Geometry: final body of the model. Coordinates: model frame, mm. A direction names the side the tool comes from. Give positions to 0.01 mm unless a question says otherwise; leave off trailing zeros. Loops run counter-clockwise (first coordinate to the right, second up) from the corner with the lowest first, then second, coordinate; pieces in that order, holes last. Notation, with made-up numbers: M 18,39 L 26,39 A23 ccw 26,69 Z; hole C -32,-28.75 d1. An arc over 180 degrees is marked long. Put each result on its own line as item: value.
```python
from build123d import *

# Parameters (mm, degrees)
ESQUISSE1_R                  = 0.85
BOSS_EXTRU_1_DEPTH           = 4
ESQUISSE2_W                  = 5
ESQUISSE2_H                  = 11.5
BOSS_EXTRU_2_DEPTH           = 21
ESQUISSE3_R                  = 1.4
ENL_V_MAT_EXTRU_1_DEPTH      = 93.33964479
CONG_1_R                     = 5
BOSS_EXTRU_3_DEPTH           = 3
BOSS_EXTRU_4_DEPTH           = 25
ESQUISSE6_R                  = 1.2
ENL_V_MAT_EXTRU_2_DEPTH      = 84.712364678
BOSS_EXTRU_6_DEPTH           = 4.5
BOSS_EXTRU_6_DEPTH_BACK      = 4
ESQUISSE9_R                  = 24
ESQUISSE9_R_2                = 21
BOSS_EXTRU_7_DEPTH           = 7
ENL_V_MAT_EXTRU_3_DEPTH      = 87.997255704
ENL_V_MAT_EXTRU_3_DEPTH_BACK = 87.997255704
ESQUISSE11_R                 = 0.9
ENL_V_MAT_EXTRU_4_DEPTH      = 87.997255704
ENL_V_MAT_EXTRU_4_DEPTH_BACK = 87.997255704
ESQUISSE12_R                 = 0.9


with BuildPart() as part:
    # Esquisse1 → Boss.-Extru.1 (new body)
    with BuildSketch(Plane.XY):
        Polygon((15.5, 18), (-15.5, 18), (-72.6, 3.278696541), (-72.6, -18), (-67.6, -18), (-67.6, -6), (-45, -6), (-45, -18), (45, -18), (45, -6), (67.6, -6), (67.6, -18), (72.6, -18), (72.6, 3.278696541), align=None)
        with Locations((-42.5, -12)):
            Circle(ESQUISSE1_R, mode=Mode.SUBTRACT)
        with Locations((-70.1, -12)):
            Circle(ESQUISSE1_R, mode=Mode.SUBTRACT)
        with Locations(Location((42.5, -12, 0), (0, 0, 180))):
            Circle(ESQUISSE1_R, mode=Mode.SUBTRACT)
        with Locations(Location((70.1, -12, 0), (0, 0, 180))):
            Circle(ESQUISSE1_R, mode=Mode.SUBTRACT)
    extrude(amount=BOSS_EXTRU_1_DEPTH)

    # Esquisse2 → Boss.-Extru.2 (add)
    with BuildSketch(Plane(origin=(0, 0, 0), x_dir=(-1, 0, 0), z_dir=(0, 0, -1))):
        with Locations((-13, 12.25)):
            Rectangle(ESQUISSE2_W, ESQUISSE2_H)
        with Locations((13, 12.25)):
            Rectangle(ESQUISSE2_W, ESQUISSE2_H)
    extrude(amount=BOSS_EXTRU_2_DEPTH)

    # Esquisse3 → Enlèv. mat.-Extru.1 (cut, through all)
    with BuildSketch(Plane.ZY.offset(15.5)):
        with Locations((-6.49, 12.25)):
            Circle(ESQUISSE3_R)
        with Locations((-14.49, 12.25)):
            Circle(ESQUISSE3_R)
    extrude(amount=-ENL_V_MAT_EXTRU_1_DEPTH, mode=Mode.SUBTRACT)

    # Congé1
    cong_1_edges = [part.edges().sort_by_distance(p)[0] for p in [
        (-15.5, 12.25, 0),
        (15.5, 12.25, 0),
    ]]
    fillet(cong_1_edges, radius=CONG_1_R)

    # Esquisse4 → Boss.-Extru.3 (add)
    with BuildSketch(Plane.XZ.offset(-6.5)):
        Polygon((-15.5, -10.5), (-39.70316927, -7.340935878), (-46.787327396, 0), (-10.5, 0), (-10.5, -10.5), align=None)
        Polygon((15.5, -10.5), (10.5, -10.5), (10.5, 0), (46.787327396, 0), (39.70316927, -7.340935878), align=None)
    extrude(amount=-BOSS_EXTRU_3_DEPTH)

    # Esquisse5 → Boss.-Extru.4 (add, through all)
    with BuildSketch(Plane.XY.offset(4)):
        Polygon((-15.466226842, 23), (-15.466226842, 18), (15.466226842, 18), (15.466226842, 23), (7.816226842, 23), (7.816226842, 28), (10.316226842, 28), (10.316226842, 30.5), (4.816226842, 30.5), (4.816226842, 26), (-4.816226842, 26), (-4.816226842, 30.5), (-10.316226842, 30.5), (-10.316226842, 28), (-7.816226842, 28), (-7.816226842, 23), align=None)
    extrude(amount=-BOSS_EXTRU_4_DEPTH)

    # Esquisse6 → Enlèv. mat.-Extru.2 (cut, through all)
    with BuildSketch(Plane.XZ.offset(-18)):
        with Locations(Location((0, -5.25, 0), (0, 0, 270))):
            Circle(ESQUISSE6_R)
        with Locations(Location((0, -15.7500125, 0), (0, 0, 270))):
            Circle(ESQUISSE6_R)
    extrude(amount=-ENL_V_MAT_EXTRU_2_DEPTH, mode=Mode.SUBTRACT)

    # Esquisse9 → Boss.-Extru.6 (add, two sides: drawn at the far end of the back side and taken through both)
    with BuildSketch(Plane(origin=(0, 0, 0), x_dir=(-1, 0, 0), z_dir=(0, 0, -1)).offset(-BOSS_EXTRU_6_DEPTH_BACK)):
        with Locations((51.15, -12)):
            Circle(ESQUISSE9_R)
        with Locations((51.15, -12)):
            Circle(ESQUISSE9_R_2, mode=Mode.SUBTRACT)
    extrude(amount=BOSS_EXTRU_6_DEPTH + BOSS_EXTRU_6_DEPTH_BACK)

    # Esquisse10 → Boss.-Extru.7 (add)
    with BuildSketch(Plane(origin=(0, 0, -4.5), x_dir=(-1, 0, 0), z_dir=(0, 0, -1))):
        with BuildLine():
            Line((27.255701517, -9.75), (30.270883639, -9.75))
            ThreePointArc((30.270883639, -9.75), (51.15, 9), (72.029116361, -9.75))
            Line((72.029116361, -9.75), (75.044298483, -9.75))
            ThreePointArc((75.044298483, -9.75), (51.15, 12), (27.255701517, -9.75))
        make_face()
        with BuildLine():
            Line((27.255701517, -14.25), (30.270883639, -14.25))
            ThreePointArc((30.270883639, -14.25), (51.15, -33), (72.029116361, -14.25))
            Line((72.029116361, -14.25), (75.044298483, -14.25))
            ThreePointArc((75.044298483, -14.25), (51.15, -36), (27.255701517, -14.25))
        make_face()
    extrude(amount=BOSS_EXTRU_7_DEPTH)

    # Esquisse11 → Enlèv. mat.-Extru.3 (cut, two sides: drawn at the far end of the back side and taken through both)
    with BuildSketch(Plane.XY.offset(4).offset(-ENL_V_MAT_EXTRU_3_DEPTH_BACK)):
        with Locations((-70.1, -12)):
            Circle(ESQUISSE11_R)
        with Locations((-42.5, -12)):
            Circle(ESQUISSE11_R)
    extrude(amount=ENL_V_MAT_EXTRU_3_DEPTH + ENL_V_MAT_EXTRU_3_DEPTH_BACK, mode=Mode.SUBTRACT)

    # Esquisse12 → Enlèv. mat.-Extru.4 (cut, two sides: drawn at the far end of the back side and taken through both)
    with BuildSketch(Plane.XY.offset(4).offset(-ENL_V_MAT_EXTRU_4_DEPTH_BACK)):
        with Locations((-71.937289482, -3.389622772)):
            Circle(ESQUISSE12_R)
        with Locations((-59.760377228, 8.787289482)):
            Circle(ESQUISSE12_R)
        with Locations((-42.539622772, 8.787289482)):
            Circle(ESQUISSE12_R)
        with Locations((-30.362710518, -3.389622772)):
            Circle(ESQUISSE12_R)
        with Locations((-30.362710518, -20.610377228)):
            Circle(ESQUISSE12_R)
        with Locations((-42.539622772, -32.787289482)):
            Circle(ESQUISSE12_R)
        with Locations((-59.760377228, -32.787289482)):
            Circle(ESQUISSE12_R)
        with Locations((-71.937289482, -20.610377228)):
            Circle(ESQUISSE12_R)
    extrude(amount=ENL_V_MAT_EXTRU_4_DEPTH + ENL_V_MAT_EXTRU_4_DEPTH_BACK, mode=Mode.SUBTRACT)


solid = part.part
```
Item 1: Pin query (flat end, axial travel): pin 1 Ø2 at (y, z) = (-9, 2.5) entering from -X; pin 2 Ø0.9 at (x, z) = (-29.5, -6.5) entering from +Y; pin 3 Ø8 at (y, z) = (22.5, -7.5) entering from +X; pin 4 Ø8 at (x, z) = (-24, -14) entering from -Y. Return the tip coordinate at first contact, or that it passes through.
Output values:
pin 1: x = -75.07
pin 2: y = 9.5
pin 3: x = 15.47
pin 4: through
Item 2: Section D-D on z = 1.5. Count the separate pieces of the cut face and the enclosed holes in it, then the cut area to 3 significant figures.
Output values:
separate pieces: 1
enclosed holes: 14
area: 4,320 mm²
Item 3: Set-up query: faces 5 (the flat face through (-74, -9.75, -8)), 6 (the flat face through (-51, -4, 0)), 7 (the flat face through (4.816, 28, -8)), 8 (the flat face through (9, 28, -8)). Return all of +Z, -Z, +X, -X, +Y, -Y with unobstructed straight access to the full face (end or side cutting, diameter ignored); none if empty.
Output values:
face 5: -Z, +X, -X
face 6: -Z
face 7: +Z, -Z, +Y
face 8: +Z, -Z, +X
Item 4: Mould query, pull axis Y, two halves, no side actions, for faces 1 (the flat face through (70, -18, 2)), 2 (the flat face through (0, 26, -8)), 3 (the cylindrical face through (12.96, 13.64, -6.67)), 4 (the flat face through (10.5, 12, -10)). Classes: pulls with the +Y half, pulls with the -Y half, needs draft (parallel to the pull), parting line crosses it, or undercut.
Output values:
face 1: pulls with the -Y half
face 2: pulls with the +Y half
face 3: undercut
face 4: needs draft
Item 5: Section C-C on x = 37. Output: boundary loops of the cut face in (y, z).
Output values:
outline: M -18,0 L 6.5,0 L 6.5,-7.69 L 9.5,-7.69 L 9.5,0 L 12.46,0 L 12.46,4 L -18,4 Z
Item 6: Line query: probe 1 along X at (y, z) = (23.5, -5.25); probe 2 along Y at (x, z) = (-17.5, -10); probe 3 along X at (y, z) = (7, -1.25). Output: solid intervals per line, ascending. Write a range as [from, to].
Output values:
probe 1: [-7.82, -1.2], [1.2, 7.82]
probe 2: [6.5, 9.5]
probe 3: [-65.81, -60.09], [-45.58, -10.5], [10.5, 45.58]
Item 7: Section B-B on x = -13. Output: boundary loops of the cut face in (y, z), then the cut area to 3 significant figures.
Output values:
outline: M -18,0 L 6.5,0 L 6.5,-21 L 23,-21 L 23,4 L -18,4 Z; hole C 12.25,-14.49 d2.8; hole C 12.25,-6.49 d2.8
area: 498 mm²
